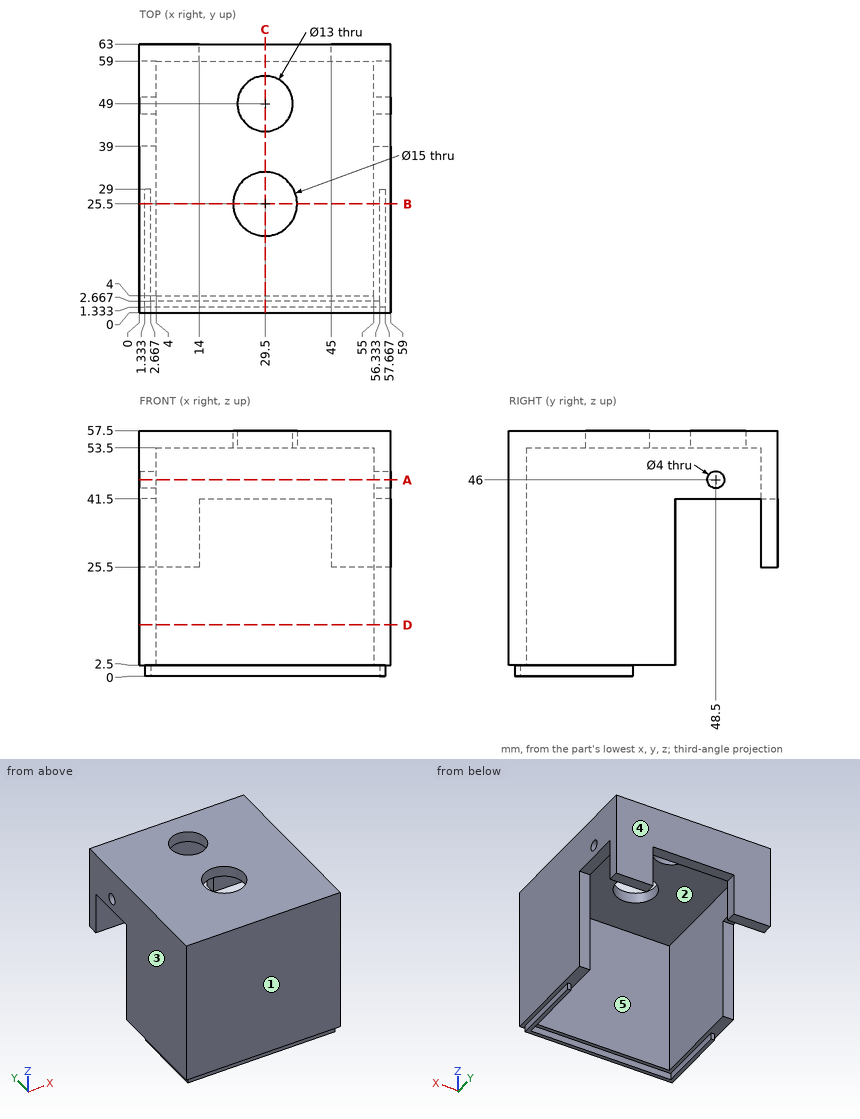
Input: dimensioned drawing with shaded views. Units: mm. Origin: part minimum x, y, z. A direction names the side the tool comes from. Round coordinates to 2 decimals unless told otherwise and drop trailing zeros. Loops run counter-clockwise (first coordinate to the right, second up) from the corner with the lowest first, then second, coordinate; pieces in that order, holes last. Notation, with made-up numbers: M 38,7.25 L 67,7.25 A14 ccw 67,34.25 Z; hole C 49,62 d3. An arc over 180 degrees is marked long. One line per question, with ' | ' between items.
(1) Material intervals for line 1 along Y through (x, z) = (29, 55); line 2 along X through (y, z) = (15, 49.5); line 3 along X through (y, z) = (25, 56), sorted ascending. Write a range as from..to.
Check result:
line 1: y = 0..18.02, 32.98..42.52, 55.48..63 | line 2: x = 0..4, 55..59 | line 3: x = 0..22.02, 36.98..59
(2) Cut plane B-B on y = 25.5. Return the cut outline in (x, z).
Check result:
outline: M 0,2.5 L 1.33,2.5 L 1.33,0 L 2.67,0 L 2.67,2.5 L 4,2.5 L 4,53.5 L 22,53.5 L 22,57.5 L 0,57.5 Z; M 37,53.5 L 55,53.5 L 55,2.5 L 56.33,2.5 L 56.33,0 L 57.67,0 L 57.67,2.5 L 59,2.5 L 59,57.5 L 37,57.5 Z
(3) Access query for the marked faces 4 and 5. Directions: +Z, -Z, +X, -X, +Y, -Y. A direction counts if a zero-diameter tool reaches every point of the face in a straight line with its end or side. Return the directions, or none.
Check result:
face 4: +Z, -Z, +X, -X, +Y | face 5: -Z
(4) Cut plane D-D on z = 12. Return the cut outline in (x, y).
Check result:
outline: M 0,0 L 59,0 L 59,39 L 55,39 L 55,4 L 4,4 L 4,39 L 0,39 Z
(5) Cut plane C-C on x = 29.5. Return the cut outline in (y, z), plus the area to 3 significant figures.
Check result:
outline: M 0,2.5 L 1.33,2.5 L 1.33,0 L 2.67,0 L 2.67,2.5 L 4,2.5 L 4,53.5 L 18,53.5 L 18,57.5 L 0,57.5 Z; M 33,53.5 L 42.5,53.5 L 42.5,57.5 L 33,57.5 Z; M 55.5,53.5 L 59,53.5 L 59,41.5 L 63,41.5 L 63,57.5 L 55.5,57.5 Z | area: 395 mm2
(6) Pull-direction query (X, two-part tool) for the marked faces 1, 2 and 3; classes: +X half, -X half, draft (parallel to the pull), parting line (faces both ways), or undercut.
Check result:
face 1: draft | face 2: undercut | face 3: -X half
(7) Contact query for flat-ended pins moving along their axis: P1, Ø1.2, axis at x = 2, y = 54, coming from the -Z side; P2, Ø1.2, axis at x = 1.5, z = 23, coming from the +Y side; P3, Ø4, axis at x = 21, y = 56, coming from the -Z side. Output: stop coordinate, or through.
Check result:
P1: stops at z = 41.5 | P2: stops at y = 39 | P3: stops at z = 53.5
(8) Cut plane A-A on z = 46. Return the cut outline in (x, y), plus the area to 3 significant figures.
Check result:
outline: M 0,0 L 59,0 L 59,46.5 L 55,46.5 L 55,4 L 4,4 L 4,46.5 L 0,46.5 Z; M 0,50.5 L 4,50.5 L 4,59 L 55,59 L 55,50.5 L 59,50.5 L 59,63 L 0,63 Z | area: 880 mm2
